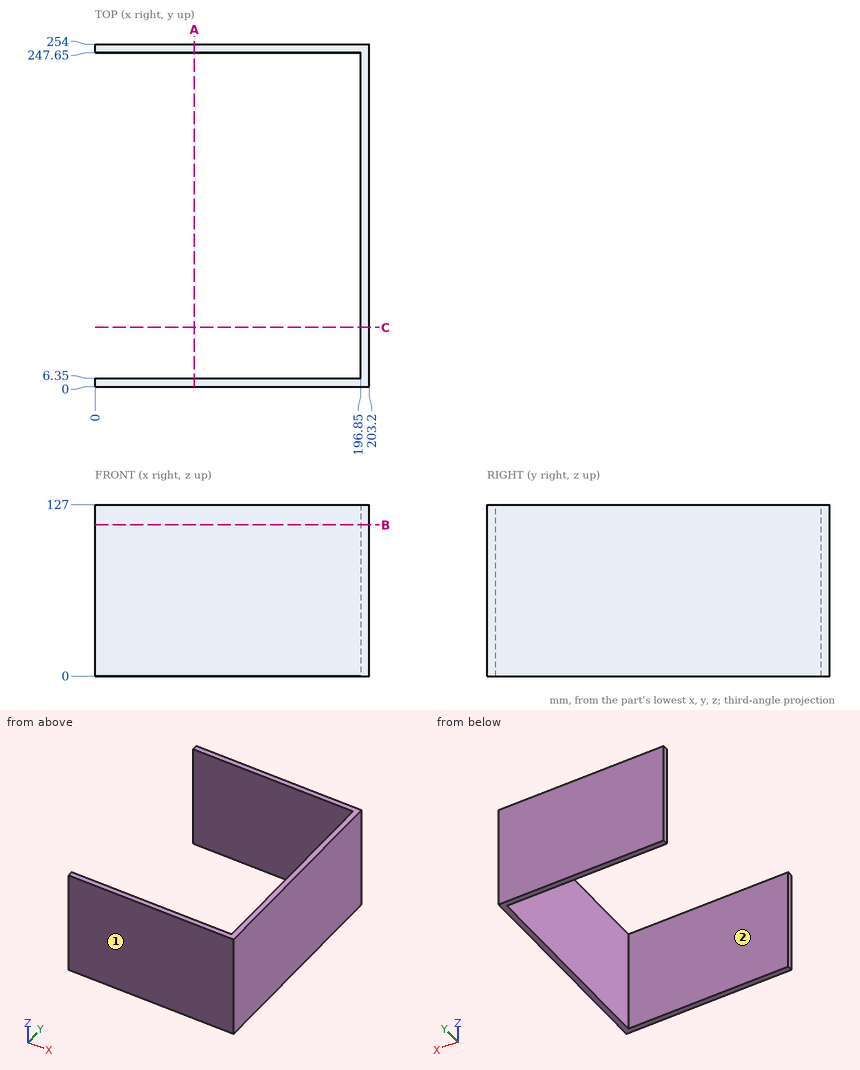
Here's the drawing with two shaded views (mm, measured from the low corner). I have some questions. A direction names the side the tool comes from. Coordinates: 2 decimals unless noted, no trailing zeros. Write each loop counter-clockwise with the first axis right and the second up, starting at its lowest first coordinate (ties: lowest second). Pieces come first, ordered by that corner, then holes. Notation, with made-up numbers: (42.25, 74) -> (83.25, 74) arc R19 ccw to (83.25, 78) -> close; hole circle Ø9 at (25, 18.25). An arc over 180 degrees is marked (long way). Use a Markdown table: item, result. Add a question column.
(1) If we section it at B-B, the plane z = 112: Write out the boundary of the cut face in (x, y).
(2) If we section it at A-A, the plane x = 73.5: Write out the boundary of the cut face in (y, z).
(3) Please list where these lines run through material, in increasing order: line 1 (Y direction, x = 174.5, z = 16.5); line 2 (X direction, y = 12.5, z = 63.5).
(4) I'm going to push a flat-ended pin straight in: P1, Ø8, axis at x = 86, z = 93, coming from the -Y side. Where does the tip first touch, or does it pass through?
(5) If we section it at C-C, the plane y = 44: Write out the boundary of the cut face in (x, z), and give its area (3 significant figures).
(6) For the marked faces 1 and 2, which set-ups out of +Z, -Z, +X, -X, +Y, -Y let a thin tool reach every point of the face, with its end or its side?
Outcome:
| question | item | result |
|---|---|---|
| 1 | outline | (0, 0) -> (203.2, 0) -> (203.2, 254) -> (0, 254) -> (0, 247.65) -> (196.85, 247.65) -> (196.85, 6.35) -> (0, 6.35) -> close |
| 2 | outline | (0, 0) -> (6.35, 0) -> (6.35, 127) -> (0, 127) -> close; (247.65, 0) -> (254, 0) -> (254, 127) -> (247.65, 127) -> close |
| 3 | line 1 | y = 0 to 6.35, 247.65 to 254 |
| 3 | line 2 | x = 196.85 to 203.2 |
| 4 | P1 | stops at y = 0 |
| 5 | outline | (196.85, 0) -> (203.2, 0) -> (203.2, 127) -> (196.85, 127) -> close |
| 5 | area | 806 mm^2 |
| 6 | face 1 | +Z, -Z, +X, -X, -Y |
| 6 | face 2 | +Z, -Z, -X |
